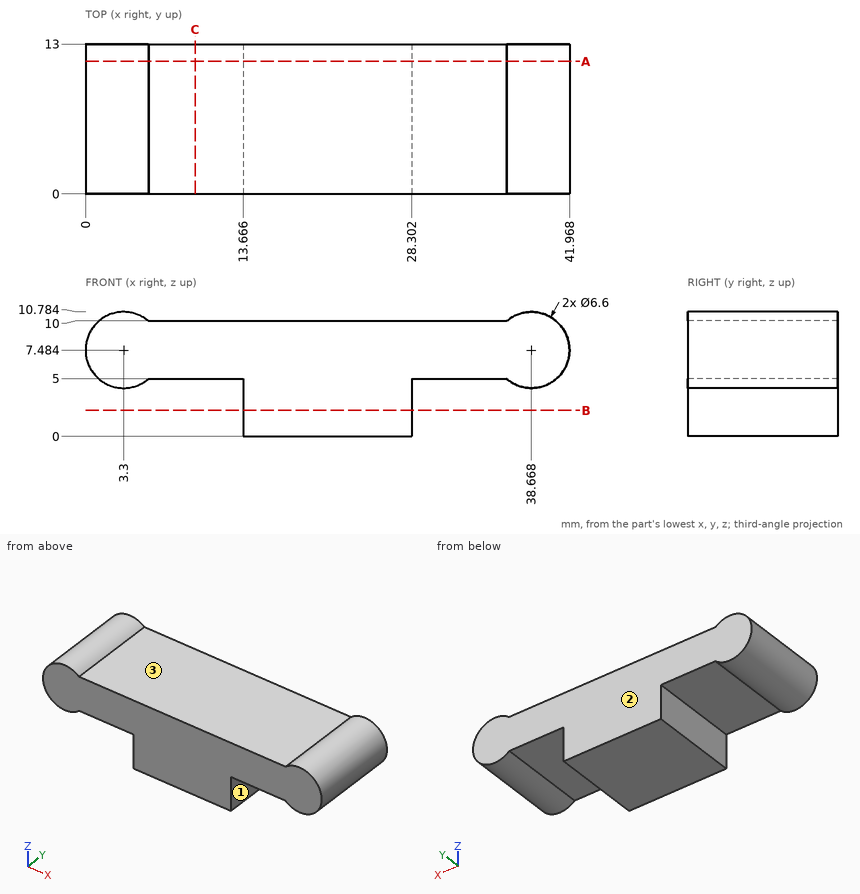
Can you work these out from the drawing? Everything is in mm from the part's minimum corner. A direction names the side the tool comes from. Give positions to 0.01 mm unless a question says otherwise; leave off trailing zeros. Loops run counter-clockwise (first coordinate to the right, second up) from the corner with the lowest first, then second, coordinate; pieces in that order, holes last. Notation, with made-up numbers: M 44.25,-15.5 L 54.25,-15.5 A29 cw 54.25,8.5 Z; hole C 18.5,28.5 d4. An arc over 180 degrees is marked long. Put each result on its own line as item: value. Start each with the question number.
(1) For the marked faces 1, 2 and 3, which set-ups out of +Z, -Z, +X, -X, +Y, -Y let a thin tool reach every point of the face, with its end or its side?
(2) Will these pins go through, and if not, where does the flat tip stop? pin 1 Ø1.5 at (x, z) = (8, 3.5) entering from -Y; pin 2 Ø4 at (y, z) = (6.5, 1.5) entering from +X; pin 3 Ø3 at (x, y) = (10.5, 3.5) entering from -Z; pin 4 Ø5 at (x, y) = (35, 5.5) entering from +Z.
(3) I want a section at C-C on x = 9.5. Please give me the cut outline in (y, z).
(4) I want a section at B-B on z = 2.25. Please give me the cut outline in (x, y).
(5) I want a section at A-A on y = 11.5. Please give me the cut outline in (x, z) (1 decimal), then the cut area to 3 significant figures.
(6) I need wall thicknesses on line 1 along X through (y, z) = (11.5, 1); line 2 along Z through (x, y) = (24, 5); line 3 along Z through (x, y) = (10.5, 11). Which ranges of each line are inside material? Lowest first, please. Write a range as [from, to].
Answer block:
1. face 1: -Z, +Y, -Y
1. face 2: +Z, -Z, +X, -X, +Y
1. face 3: +Z, +Y, -Y
2. pin 1: through
2. pin 2: x = 28.3
2. pin 3: z = 5
2. pin 4: z = 10.57
3. outline: M 0,5 L 13,5 L 13,10 L 0,10 Z
4. outline: M 13.67,0 L 28.3,0 L 28.3,13 L 13.67,13 Z
5. outline: M 5.4,10 A3.3 ccw long 5.5,5 L 13.7,5 L 13.7,0 L 28.3,0 L 28.3,5 L 36.5,5 A3.3 ccw long 36.5,10 Z
5. area: 289 mm^2
6. line 1: [13.67, 28.3]
6. line 2: [0, 10]
6. line 3: [5, 10]
